Read the model definition and answer for the solid it produces. Units are mm, in the model's axes. A direction names the side the tool comes from. Coordinates: 2 decimals unless noted, no trailing zeros. Loops run counter-clockwise (first coordinate to the right, second up) from the corner with the lowest first, then second, coordinate; pieces in that order, holes last. Notation, with made-up numbers: (25.5, 71) -> (43.5, 71) arc R17 ccw to (43.5, 89) -> close; hole circle Ø6 at (37, -11). An arc over 180 degrees is marked (long way). Answer as a JSON object with one key per item and string values. Group by question number.
Q1. For faces 4 (the flat face through (3.796, -22.083, -20.41)), 5 (the cylindrical face through (-14.3, -17.3, -25.6)), 6 (the flat face through (11.9, -20.47, -45.57)), determine the directions among +Z, -Z, +X, -X, +Y, -Y from which every point of the face is accessible in a straight line to the end or side of a thin tool.
Q2. Determine the mould class of faces 1 (the flat face through (-12.53, -21.55, -20.41)), 2 (the flat face through (19.48, 7.2, -45.57)), 3 (the flat face through (-8, -12.837, 1)) for opening direction X: released by +X, released by -X, zero draft, split by the parting line, or undercut.
Q3. Each of these flat-tipped pins is pushed along its axis until it touches: P1, Ø10.5, axis at y = 2, z = -47.5, coming from the +X side; P2, Ø10, axis at y = -13, z = -48, coming from the +X side; P3, Ø7, axis at y = -14.5, z = -23.5, coming from the +X side. Where does it stop, or does it pass through?
Q4. The part is cut by section A-A on z = -25.5. State how many separate pieces and enclosed holes the cut face has, and give its area (3 significant figures).
Q5. Straight lines are drawn through the part: line 1 along Y through (x, z) = (0, -32); line 2 along X through (y, z) = (0, -35); line 3 along X through (y, z) = (3, -10.5). For each, find the intervals that lie inside material, in ascending order. Write a range as [from, to].
Q6. The part is cut by section B-B on y = 2. Write down the section's boundary in (x, z).
from build123d import *

# Parameters (mm, degrees)
SKETCH2_W           = 6
SKETCH2_H           = 1
BOSS_EXTRUDE1_DEPTH = 2.25
BOSS_EXTRUDE2_START = -50.5
BOSS_EXTRUDE2_DEPTH = 50.5
SKETCH2_5_R         = 5.656929669
CUT_EXTRUDE1_DEPTH  = 0.25
FILLET1_R           = 2
CUT_EXTRUDE3_DEPTH  = 10


# Read off the part's stored shape, not the designer's step: Boss-Extrude2
with BuildPart() as part:
    # Sketch2 → Boss-Extrude1 (new body)
    with BuildSketch(Plane.XY):
        Polygon((17.226279442, -9.945597073), (24.926279442, -5.5), (24.926279442, 5.5), (15.4, 11), (7.7, 6.554402927), (0, 11), (-9.526279442, 5.5), (-9.526279442, -3.391194146), (-17.226279442, -7.836791218), (-17.226279442, -18.836791218), (-7.7, -24.336791218), (0, -19.891194146), (7.7, -24.336791218), (17.226279442, -18.836791218), align=None)
        with Locations((-7.698015444, -13.337039288)):
            Rectangle(SKETCH2_W, SKETCH2_H, mode=Mode.SUBTRACT)
        with Locations((7.7, -13.336791218)):
            Rectangle(SKETCH2_W, SKETCH2_H, mode=Mode.SUBTRACT)
        Rectangle(SKETCH2_W, SKETCH2_H, mode=Mode.SUBTRACT)
        with Locations((15.401984556, 0.000248069)):
            Rectangle(SKETCH2_W, SKETCH2_H, mode=Mode.SUBTRACT)
    extrude(amount=BOSS_EXTRUDE1_DEPTH)

    # Boss-Extrude2 outline → Boss-Extrude2 (add)
    # profile 1 of 3: a face of its own
    with BuildSketch(Plane.XY.offset(BOSS_EXTRUDE2_START)):
        Polygon((17.226279442, -9.945597073), (24.926279442, -5.5), (24.926279442, 5.5), (15.4, 11), (7.7, 6.554402927), (0, 11), (-9.526279442, 5.5), (-9.526279442, -3.391194146), (-17.226279442, -7.836791218), (-17.226279442, -18.836791218), (-7.7, -24.336791218), (0, -19.891194146), (7.7, -24.336791218), (17.226279442, -18.836791218), align=None)
        with BuildLine():
            ThreePointArc((13.743882842, -8.565891912), (11.540567195, -20.010623971), (0.538311185, -16.165256053))
            Line((0.538311185, -16.165256053), (-0.538311185, -16.165256053))
            ThreePointArc((-0.538311185, -16.165256053), (-14.438217046, -17.063241411), (-6.288758272, -5.767220769))
            Line((-6.288758272, -5.767220769), (-5.82928192, -5.030852045))
            ThreePointArc((-5.82928192, -5.030852045), (-3.985729856, 6.588167994), (7.161688815, 2.828464835))
            Line((7.161688815, 2.828464835), (8.238311185, 2.828464835))
            ThreePointArc((8.238311185, 2.828464835), (22.062914613, 3.859477797), (14.290341933, -7.619623283))
            Line((14.290341933, -7.619623283), (13.743882842, -8.565891912))
        make_face(mode=Mode.SUBTRACT)
    # profile 2 of 3: a face of its own
    with BuildSketch(Plane.XY.offset(BOSS_EXTRUDE2_START)):
        with BuildLine():
            ThreePointArc((6.325009737, -5.760551929), (7.7, -5.636791218), (9.074990263, -5.760551929))
            Line((9.074990263, -5.760551929), (9.526279442, -5.5))
            Line((9.526279442, -5.5), (9.526279442, -4.978896143))
            ThreePointArc((9.526279442, -4.978896143), (8.731604391, -3.85), (8.151289178, -2.597343147))
            Line((8.151289178, -2.597343147), (7.7, -2.336791218))
            Line((7.7, -2.336791218), (7.248710822, -2.597343147))
            ThreePointArc((7.248710822, -2.597343147), (6.668395609, -3.85), (5.873720558, -4.978896143))
            Line((5.873720558, -4.978896143), (5.873720558, -5.5))
            Line((5.873720558, -5.5), (6.325009737, -5.760551929))
        make_face()
    # profile 3 of 3: a face of its own
    with BuildSketch(Plane.XY.offset(BOSS_EXTRUDE2_START)):
        with BuildLine():
            ThreePointArc((0.451289178, -10.739448071), (1.031604391, -9.486791218), (1.826279442, -8.357895075))
            Line((1.826279442, -8.357895075), (1.826279442, -7.836791218))
            Line((1.826279442, -7.836791218), (1.374990263, -7.57623929))
            ThreePointArc((1.374990263, -7.57623929), (0, -7.7), (-1.374990263, -7.57623929))
            Line((-1.374990263, -7.57623929), (-1.826279442, -7.836791218))
            Line((-1.826279442, -7.836791218), (-1.826279442, -8.357895075))
            ThreePointArc((-1.826279442, -8.357895075), (-1.031604391, -9.486791218), (-0.451289178, -10.739448071))
            Line((-0.451289178, -10.739448071), (0, -11))
            Line((0, -11), (0.451289178, -10.739448071))
        make_face()
    extrude(amount=BOSS_EXTRUDE2_DEPTH)

    # Sketch2_5 → Cut-Extrude1 (cut)
    with BuildSketch(Plane.XY):
        with Locations(Location((15.4, 0, 0), (0, 0, 180))):
            Circle(SKETCH2_5_R)
        Circle(SKETCH2_5_R)
        with Locations((7.7, -13.336791218)):
            Circle(SKETCH2_5_R)
        with Locations(Location((-7.7, -13.336791218, 0), (0, 0, 180))):
            Circle(SKETCH2_5_R)
    extrude(amount=CUT_EXTRUDE1_DEPTH, mode=Mode.SUBTRACT)

    # Fillet1
    fillet1_edges = [part.edges().sort_by_distance(p)[0] for p in [
        (20.163139721, 8.25, 2.25),
        (11.55, 8.777201464, 2.25),
        (24.926279442, 0, 2.25),
        (21.076279442, -7.722798536, 2.25),
        (3.85, 8.777201464, 2.25),
        (-9.526279442, 1.054402927, 2.25),
        (-4.763139721, 8.25, 2.25),
        (-3.85, -22.113992682, 2.25),
        (-13.376279442, -5.613992682, 2.25),
        (-17.226279442, -13.336791218, 2.25),
        (-12.463139721, -21.586791218, 2.25),
        (17.226279442, -14.391194146, 2.25),
        (12.463139721, -21.586791218, 2.25),
        (3.85, -22.113992682, 2.25),
    ]]
    fillet(fillet1_edges, radius=FILLET1_R)

    # Sketch7 → Cut-Extrude3 (cut)
    with BuildSketch(Plane(origin=(0, 0, -50.5), x_dir=(-1, 0, 0), z_dir=(0, 0, -1))):
        Polygon((-7.7, -24.336791218), (0, -19.891194146), (7.7, -24.336791218), (17.226279442, -18.836791218), (17.226279442, -7.836791218), (9.526279442, -3.391194146), (9.526279442, 5.5), (0, 11), (-7.7, 6.554402927), (-15.4, 11), (-24.926279442, 5.5), (-24.926279442, -5.5), (-17.226279442, -9.945597073), (-17.226279442, -18.836791218), align=None)
        Polygon((-7.7, 5.111027254), (-15.4, 9.556624327), (-23.676279442, 4.778312164), (-23.676279442, -4.778312164), (-15.976279442, -9.223909236), (-15.976279442, -18.115103382), (-7.7, -22.893415545), (0, -18.447818473), (7.7, -22.893415545), (15.976279442, -18.115103382), (15.976279442, -8.558479055), (8.276279442, -4.112881982), (8.276279442, 4.778312164), (0, 9.556624327), align=None, mode=Mode.SUBTRACT)
    extrude(amount=-CUT_EXTRUDE3_DEPTH, mode=Mode.SUBTRACT)


solid = part.part
Final values:
{
 "1": {"face 4": "+Z, -Z, -Y", "face 5": "-Z", "face 6": "-Z, +X, -Y"},
 "2": {"face 1": "released by -X", "face 2": "released by +X", "face 3": "undercut"},
 "3": {"P1": "stops at x = 23.68", "P2": "stops at x = 18.1", "P3": "stops at x = 17.23"},
 "4": {"separate pieces": "3", "enclosed holes": "1", "area": "308 mm2"},
 "5": {"line 1": "y = [-19.89, -16.17], [-11, -7.7], [7.7, 11]", "line 2": "x = [-9.53, -7.7], [23.1, 24.93]", "line 3": "x = [-9.53, -7.09], [7.09, 8.31], [22.49, 24.93]"},
 "6": {"outline": "(-9.53, -40.5) -> (-8.28, -40.5) -> (-8.28, -50.5) -> (-7.44, -50.5) -> (-7.44, 0) -> (-5.29, 0) -> (-5.29, 0.25) -> (5.29, 0.25) -> (5.29, 0) -> (10.11, 0) -> (10.11, 0.25) -> (20.69, 0.25) -> (20.69, 0) -> (22.84, 0) -> (22.84, -50.5) -> (23.68, -50.5) -> (23.68, -40.5) -> (24.93, -40.5) -> (24.93, 0.25) arc R2 ccw to (22.93, 2.25) -> (-7.53, 2.25) arc R2 ccw to (-9.53, 0.25) -> close"}
}
